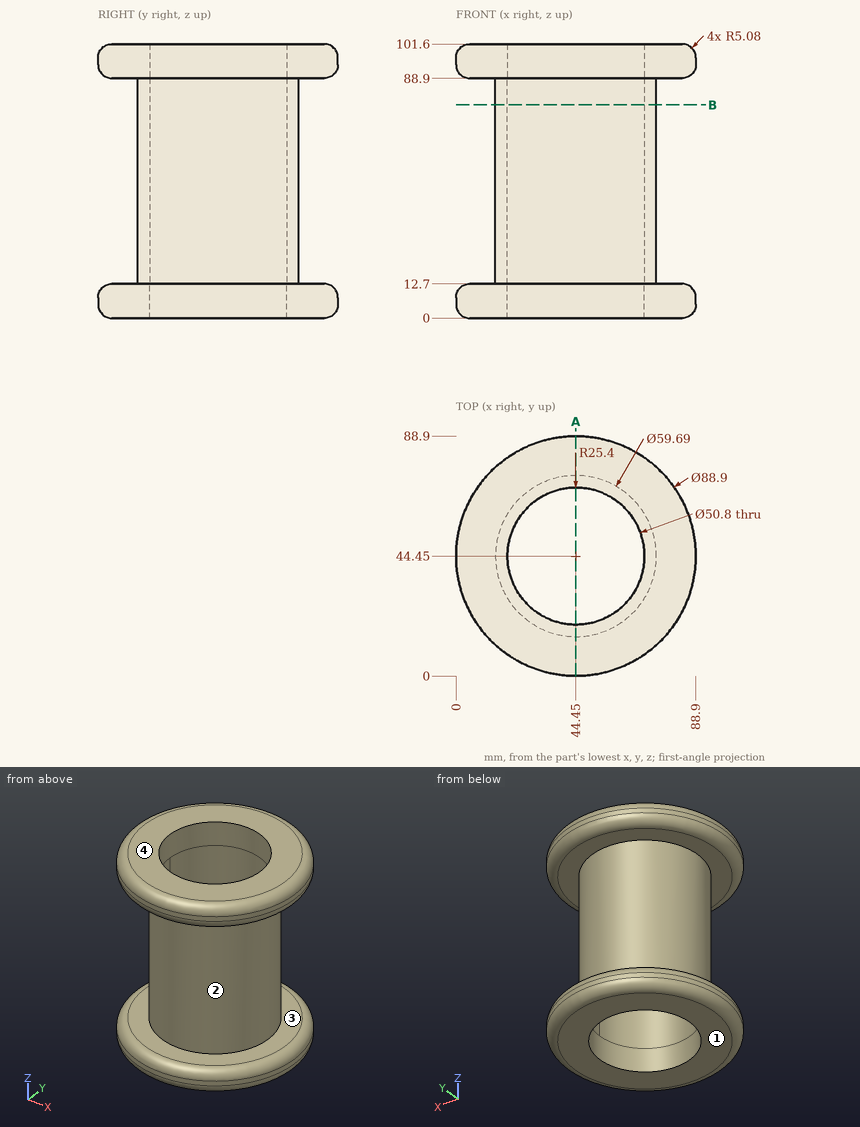
Could you check a few things on this drawing? It's one solid part, dimensions in mm from its lowest x, y, z. Coordinates: 2 decimals unless noted, no trailing zeros. Order: outer loops, then holes, each group sorted by start corner. A loop starts at its lowest first (then second) coordinate and runs counter-clockwise, first axis right, second up. Notation, with made-up numbers: (86, 21) -> (96, 21) arc R28 ccw to (96, 53) -> close; hole circle Ø10 at (2.25, 1.5). An arc over 180 degrees is marked (long way). Answer in a Markdown table with one row per item.
(1) Will these pins go through, and if not, where does the flat tip stop? pin 1 Ø2 at (x, z) = (39.5, 34.5) entering from +Y; pin 2 Ø12 at (x, z) = (33, 47) entering from +Y; pin 3 Ø10 at (x, z) = (38, 56) entering from +Y.
Answer key:
| item | result |
|---|---|
| pin 1 | y = 74.03 |
| pin 2 | y = 73.79 |
| pin 3 | y = 74.26 |
(2) I want a section at B-B on z = 79. List the corners of the cut face in (x, y) for me (3 decimals).
Answer key:
| item | result |
|---|---|
| outline | circle Ø59.69 at (44.45, 44.45); hole circle Ø50.8 at (44.45, 44.45) |
(3) Thinking about a two-plate mould opening in Z: for the marked faces 1, 2, 3 and 4, which applies, +Z half, -Z half, draft (parallel to the pull), parting line (faces both ways), or undercut?
Answer key:
| item | result |
|---|---|
| face 1 | -Z half |
| face 2 | undercut |
| face 3 | undercut |
| face 4 | +Z half |
(4) I want a section at A-A on x = 44.45. List the corners of the cut face in (y, z) for me (3 decimals).
Answer key:
| item | result |
|---|---|
| outline | (0, 5.08) arc R5.08 ccw to (5.08, 0) -> (19.05, 0) -> (19.05, 101.6) -> (5.08, 101.6) arc R5.08 ccw to (0, 96.52) -> (0, 93.98) arc R5.08 ccw to (5.08, 88.9) -> (14.605, 88.9) -> (14.605, 12.7) -> (5.08, 12.7) arc R5.08 ccw to (0, 7.62) -> close; (69.85, 0) -> (83.82, 0) arc R5.08 ccw to (88.9, 5.08) -> (88.9, 7.62) arc R5.08 ccw to (83.82, 12.7) -> (74.295, 12.7) -> (74.295, 88.9) -> (83.82, 88.9) arc R5.08 ccw to (88.9, 93.98) -> (88.9, 96.52) arc R5.08 ccw to (83.82, 101.6) -> (69.85, 101.6) -> close |
(5) Please list where these lines run through material, in increasing order: probe 1 along Y at (x, z) = (44.45, 96.75); probe 2 along Z at (x, y) = (79.5, 50.5); probe 3 along Y at (x, z) = (44.45, 92.5).
Answer key:
| item | result |
|---|---|
| probe 1 | 0.01 to 19.05, 69.85 to 88.89 |
| probe 2 | 0 to 12.7, 88.9 to 101.6 |
| probe 3 | 0.22 to 19.05, 69.85 to 88.68 |
